Can you work these out from the model? Positions are in its coordinate system, mm. Face numbers are marked on the shaded views. A direction names the side the tool comes from. Round coordinates to 2 decimals unless told otherwise and drop trailing zeros. Loops run counter-clockwise (first coordinate to the right, second up) from the corner with the lowest first, then second, coordinate; pieces in that order, holes last. Notation, with made-up numbers: (-7.5, 15) - (26.5, 15) arc R14 cw to (26.5, 25) - close; hole circle Ø4 at (52.5, -33.75). An arc over 180 degrees is marked (long way). Answer as CSV lines item,"result".
Autodesk Fusion 360 part; units mm, degrees
sketch "Sketch1" plane through (0, 0, 0) normal (0, 0, 1) x (1, 0, 0) in component "Motor v2"
  circle A0 centre (0, 0) radius 12.25
  circle A1 centre (0, 0) radius 3.5
  circle A2 centre (0, 0) radius 2
  dimension "d1_2_1_1_1" = 24.5
  dimension "d8_1_1_1_1" = 7
  dimension "d9_1_1_1_1" = 4
  dimension "d478_1_1" = 0
  dimension "d479_1_1" = 0
  dimension "d480_1_1" = 0
  dimension "d481_1_1" = 0
ref_plane "WorkPlane1" through (0, 0, -23) normal (0, 0, 1) x (1, 0, 0) in component "Motor v2"
sketch "Sketch2" plane through (0, 0, -23) normal (0, 0, 1) x (1, 0, 0) in component "Motor v2"
  circle A0 centre (0, 0) radius 11.75
  dimension "d3_3_1_1" = 23.5
extrude "Extrude1" add sketch "Sketch1" against normal blind 23 contours A0 | A1 | A2 in component "Motor v2"
extrude "Extrude2" add sketch "Sketch2" against normal blind 31 in component "Motor v2"
extrude "Extrude3" add sketch "Sketch1" along normal blind 3 contours A1 | A2 in component "Motor v2"
extrude "Extrude4" add sketch "Sketch1" along normal blind 10 contours A2 in component "Motor v2"
component "Motor v2" placed x (1, 0, 0) y (0, 1, 0) z (0, 0, 1) at (0, 0, 0)
equation "d1_2_1_1_1 = 23.5 mm + 1 mm"
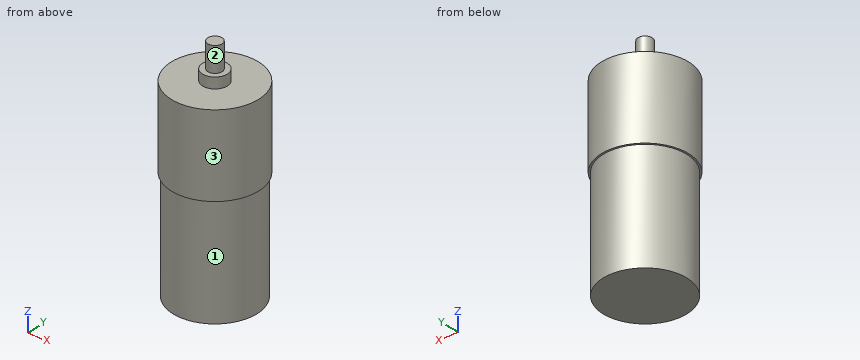
Q1. Imagine slicing it at A-A (x = 0). Write out the boundary of the cut face in (y, z).
Checks:
outline,"(-12.25, -23) - (-11.75, -23) - (-11.75, -54) - (11.75, -54) - (11.75, -23) - (12.25, -23) - (12.25, 0) - (3.5, 0) - (3.5, 3) - (2, 3) - (2, 10) - (-2, 10) - (-2, 3) - (-3.5, 3) - (-3.5, 0) - (-12.25, 0) - close"
Q2. On a 3-axis mill with a long thin cutter (end or side, diameter ignored), from which of +Z, -Z, +X, -X, +Y, -Y can I reach the whole of each face in a straight line? I mean the marked faces 1, 2 and 3. Say none if no direction works.
Checks:
face 1,"-Z"
face 2,"+Z"
face 3,"+Z, -Z"
Q3. If I drill on line 1 along Z through (x, y) = (0, -3.25); line 2 along Z through (x, y) = (5.5, 2.5); line 3 along Y through (x, z) = (0.5, -38), over which ranges is the centre line in solid material (lowest first)? Write a range as [from, to].
Checks:
line 1,"[-54, 3]"
line 2,"[-54, 0]"
line 3,"[-11.74, 11.74]"
Q4. I'm going to push flat-ended pins straight in: pin 1 Ø8 at (x, z) = (3, -28) entering from +Y; pin 2 Ø12 at (x, y) = (-9, 7) entering from +Z; pin 3 Ø12 at (x, z) = (9, -19) entering from -Y. Where does each tip first touch, or does it pass through?
Checks:
pin 1,"y = 11.75"
pin 2,"z = 0"
pin 3,"y = -11.88"
Q5. Imagine slicing it at C-C (z = 4.5). Write out the boundary of the cut face in (x, y), then the cut area to 3 significant figures.
Checks:
outline,"circle Ø4 at (0, 0)"
area,"12.6 mm²"
Q6. Imagine slicing it at D-D (x = -10). Write out the boundary of the cut face in (y, z), then the cut area to 3 significant figures.
Checks:
outline,"(-7.08, -23) - (-6.17, -23) - (-6.17, -54) - (6.17, -54) - (6.17, -23) - (7.08, -23) - (7.08, 0) - (-7.08, 0) - close"
area,"708 mm²"
